Model file for the job. Use its own axes, mm. Face numbers are marked on the shaded views. A direction names the side the tool comes from. Give positions to 0.01 mm unless a question says otherwise; leave off trailing zeros. Loops run counter-clockwise (first coordinate to the right, second up) from the corner with the lowest first, then second, coordinate; pieces in that order, holes last. Notation, with made-up numbers: (61.5, 59.25) - (69.5, 59.25) arc R19 cw to (69.5, 71.25) - close; hole circle Ø3 at (-10, 61.5). An arc over 180 degrees is marked (long way). Use a Markdown table: item, result.
from build123d import *

# Parameters (mm, degrees)
ESBO_O1_W                                   = 75
ESBO_O1_H                                   = 30
RESSALTO_EXTRUS_O1_DEPTH                    = 10.7
ESBO_O2_R                                   = 6
CORTE_EXTRUS_O1_DEPTH                       = 10
ESBO_O7_R                                   = 11
CORTE_EXTRUS_O6_DEPTH                       = 7
FURO_ROSCADO_PARA_CONDU_TE_DE_1_4_281_D     = 6.6294
FURO_ROSCADO_PARA_CONDU_TE_DE_1_4_281_DEPTH = 15
FURO_ROSCADO_PARA_CONDU_TE_DE_1_4_281_TIP   = 1.991672694
FURO_ROSCADO_PARA_CONDU_TE_DE_1_4_282_D     = 6.6294
FURO_ROSCADO_PARA_CONDU_TE_DE_1_4_282_DEPTH = 14.96
FURO_ROSCADO_PARA_CONDU_TE_DE_1_4_282_TIP   = 1.991672694
FURO_ROSCADO_PARA_CONDU_TE_DE_1_4_283_D     = 6.6294
FURO_ROSCADO_PARA_CONDU_TE_DE_1_4_283_DEPTH = 15
FURO_ROSCADO_PARA_CONDU_TE_DE_1_4_283_TIP   = 1.991672694
FURO_ROSCADO_PARA_CONDU_TE_DE_1_4_284_D     = 6.6294
FURO_ROSCADO_PARA_CONDU_TE_DE_1_4_284_DEPTH = 12
FURO_ROSCADO_PARA_CONDU_TE_DE_1_4_284_TIP   = 1.991672694


with BuildPart() as part:
    # Esboço1 → Ressalto-extrusão1 (new body)
    with BuildSketch(Plane.XY):
        Rectangle(ESBO_O1_W, ESBO_O1_H)
    extrude(amount=RESSALTO_EXTRUS_O1_DEPTH)

    # Esboço2 → Corte-extrusão1 (cut)
    with BuildSketch(Plane.XY.offset(10.7)):
        with Locations((-24, 0)):
            Circle(ESBO_O2_R)
        with Locations((24, 0)):
            Circle(ESBO_O2_R)
    extrude(amount=-CORTE_EXTRUS_O1_DEPTH, mode=Mode.SUBTRACT)

    # Esboço7 → Corte-extrusão6 (cut)
    with BuildSketch(Plane.XY.offset(10.7)):
        Circle(ESBO_O7_R)
    extrude(amount=-CORTE_EXTRUS_O6_DEPTH, mode=Mode.SUBTRACT)

    # Furo roscado para conduíte de 1/4-281
    with Locations(Plane(origin=(0, 15, 0), x_dir=(1, 0, 0), z_dir=(0, 1, 0))):
        with Locations((-24, -5.35), (24, -5.35)):
            Hole(FURO_ROSCADO_PARA_CONDU_TE_DE_1_4_281_D / 2, depth=FURO_ROSCADO_PARA_CONDU_TE_DE_1_4_281_DEPTH)
            with Locations((0, 0, -(FURO_ROSCADO_PARA_CONDU_TE_DE_1_4_281_DEPTH + FURO_ROSCADO_PARA_CONDU_TE_DE_1_4_281_TIP / 2))):  # 118° drill point
                Cone(0, FURO_ROSCADO_PARA_CONDU_TE_DE_1_4_281_D / 2, FURO_ROSCADO_PARA_CONDU_TE_DE_1_4_281_TIP, mode=Mode.SUBTRACT)

    # Furo roscado para conduíte de 1/4-282
    with Locations(Plane.ZY.offset(37.5)):
        with Locations((5.35, 0)):
            Hole(FURO_ROSCADO_PARA_CONDU_TE_DE_1_4_282_D / 2, depth=FURO_ROSCADO_PARA_CONDU_TE_DE_1_4_282_DEPTH)
            with Locations((0, 0, -(FURO_ROSCADO_PARA_CONDU_TE_DE_1_4_282_DEPTH + FURO_ROSCADO_PARA_CONDU_TE_DE_1_4_282_TIP / 2))):  # 118° drill point
                Cone(0, FURO_ROSCADO_PARA_CONDU_TE_DE_1_4_282_D / 2, FURO_ROSCADO_PARA_CONDU_TE_DE_1_4_282_TIP, mode=Mode.SUBTRACT)

    # Furo roscado para conduíte de 1/4-283
    with Locations(Plane(origin=(37.5, 0, 0), x_dir=(0, 0, -1), z_dir=(1, 0, 0))):
        with Locations((-5.35, 0)):
            Hole(FURO_ROSCADO_PARA_CONDU_TE_DE_1_4_283_D / 2, depth=FURO_ROSCADO_PARA_CONDU_TE_DE_1_4_283_DEPTH)
            with Locations((0, 0, -(FURO_ROSCADO_PARA_CONDU_TE_DE_1_4_283_DEPTH + FURO_ROSCADO_PARA_CONDU_TE_DE_1_4_283_TIP / 2))):  # 118° drill point
                Cone(0, FURO_ROSCADO_PARA_CONDU_TE_DE_1_4_283_D / 2, FURO_ROSCADO_PARA_CONDU_TE_DE_1_4_283_TIP, mode=Mode.SUBTRACT)

    # Furo roscado para conduíte de 1/4-284
    with Locations(Plane(origin=(0, -15, 0), x_dir=(-1, 0, 0), z_dir=(0, -1, 0))):
        with Locations((15, -5.35), (-15, -5.35)):
            Hole(FURO_ROSCADO_PARA_CONDU_TE_DE_1_4_284_D / 2, depth=FURO_ROSCADO_PARA_CONDU_TE_DE_1_4_284_DEPTH)
            with Locations((0, 0, -(FURO_ROSCADO_PARA_CONDU_TE_DE_1_4_284_DEPTH + FURO_ROSCADO_PARA_CONDU_TE_DE_1_4_284_TIP / 2))):  # 118° drill point
                Cone(0, FURO_ROSCADO_PARA_CONDU_TE_DE_1_4_284_D / 2, FURO_ROSCADO_PARA_CONDU_TE_DE_1_4_284_TIP, mode=Mode.SUBTRACT)


solid = part.part
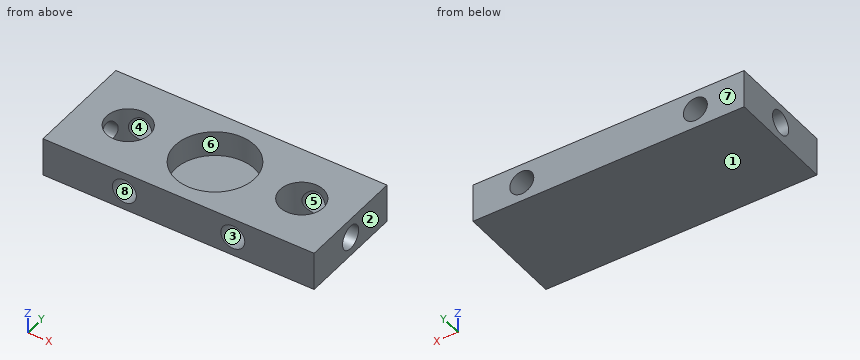
(1) Drill centre lines: probe 1 along Z at (x, y) = (-15, -11.75); probe 2 along X at (y, z) = (-1.5, 5.5); probe 3 along X at (y, z) = (-11.5, 3.5). Where is each one in solid material? Low to high. Write a range as [from, to].
Computed:
| item | result |
|---|---|
| probe 1 | [0, 2.04], [8.66, 10.7] |
| probe 2 | [-18.19, -15.8], [-14.2, -10.9], [10.9, 14.2], [15.8, 18.19] |
| probe 3 | [-37.5, -17.75], [-12.25, 12.25], [17.75, 37.5] |
(2) 3-axis set-ups, long thin cutter, end or side, ignore diameter. For the marked faces 5, 6, 7 and 8: which of +Z, -Z, +X, -X, +Y, -Y reach the whole face in a straight line?
Computed:
| item | result |
|---|---|
| face 5 | +Y |
| face 6 | +Z |
| face 7 | +Z, -Z, +X, -X, +Y |
| face 8 | -Y |
(3) Pin check, flat tips, straight feed: P1, Ø1.5, axis at x = 4.5, y = 8, coming from the +Z side; P2, Ø4, axis at x = 24, z = 5.35, coming from the +Y side; P3, Ø6, axis at x = 15, z = 5.35, coming from the -Y side. Stop position of each tip, or through.
Computed:
| item | result |
|---|---|
| P1 | z = 3.7 |
| P2 | y = -5.66 |
| P3 | y = -2.81 |
(4) Slice it at C-C, the plane x = 0. Write the cut outline in (y, z), plus the area to 3 significant figures.
Computed:
| item | result |
|---|---|
| outline | (-15, 0) - (15, 0) - (15, 10.7) - (11, 10.7) - (11, 3.7) - (-11, 3.7) - (-11, 10.7) - (-15, 10.7) - close |
| area | 167 mm² |
(5) Slice it at B-B, the plane y = 0. Write the cut outline in (x, z), plus the area to 3 significant figures.
Computed:
| item | result |
|---|---|
| outline | (-37.5, 0) - (37.5, 0) - (37.5, 2.04) - (30, 2.04) - (30, 0.7) - (18, 0.7) - (18, 10.7) - (11, 10.7) - (11, 3.7) - (-11, 3.7) - (-11, 10.7) - (-18, 10.7) - (-18, 0.7) - (-30, 0.7) - (-30, 2.04) - (-37.5, 2.04) - close; (-37.5, 8.66) - (-30, 8.66) - (-30, 10.7) - (-37.5, 10.7) - close; (30, 8.66) - (37.5, 8.66) - (37.5, 10.7) - (30, 10.7) - close |
| area | 309 mm² |
(6) Slice it at A-A, the plane x = -24. Write the cut outline in (y, z).
Computed:
| item | result |
|---|---|
| outline | (-15, 0) - (15, 0) - (15, 2.04) - (6, 2.04) - (6, 0.7) - (-6, 0.7) - (-6, 10.7) - (-15, 10.7) - close; (6, 8.66) - (15, 8.66) - (15, 10.7) - (6, 10.7) - close |
(7) Slice it at D-D, the plane y = -12. Write the cut outline in (x, z).
Computed:
| item | result |
|---|---|
| outline | (-37.5, 0) - (37.5, 0) - (37.5, 10.7) - (-37.5, 10.7) - close; hole circle Ø6.63 at (-15, 5.35); hole circle Ø6.63 at (15, 5.35) |
(8) Mould opens along Z. For the marked faces 1, 2, 3 and 4 say: pulls with the +Z half, pulls with the -Z half, needs draft (parallel to the pull), parting line crosses it, or undercut.
Computed:
| item | result |
|---|---|
| face 1 | pulls with the -Z half |
| face 2 | needs draft |
| face 3 | undercut |
| face 4 | undercut |
